```python
from build123d import *

# Parameters (mm, degrees)
F0_R     = 9.5
F0_R_2   = 4.1
F0_R_3   = 1.9
F1_DEPTH = 2
F2_R     = 4.1
F2_R_2   = 1.9
F3_DEPTH = 5.5
F4_R     = 1.5
F7_DEPTH = 7


# Not quite as in the source:
# - a feature names something its author has since deleted; it is built from what else it names


with BuildPart() as f1:
    # F0 (on Top) → F1 (new body)
    with BuildSketch(Plane.XY):
        Circle(F0_R)
        Circle(F0_R_2, mode=Mode.SUBTRACT)
        Circle(F0_R_2)
        Circle(F0_R_3, mode=Mode.SUBTRACT)
        Circle(F0_R_3)
    extrude(amount=F1_DEPTH)

    # F2 (on Top) → F3 (join)
    with BuildSketch(Plane.XY):
        Circle(F2_R)
        Circle(F2_R_2, mode=Mode.SUBTRACT)
    extrude(amount=F3_DEPTH)

    # F4
    f4_edges = [f1.edges().sort_by_distance(p)[0] for p in [
        (-9.5, 0, 0),
    ]]
    fillet(f4_edges, radius=F4_R)

    # F5 (on Front) → F6 (revolve, cut)
    with BuildSketch(Plane.XZ):
        with BuildLine():
            ThreePointArc((0, 0), (23.1570723538, -9.489364109), (32.9962119038, -32.5))
            ThreePointArc((32.9962119038, -32.5), (23.510635891, -8.8429276462), (0, 1))
            Line((0, 1), (0, 0))
        make_face()
    revolve(axis=Axis((0, 0, -31.5146126637), (0, 0, -1)), mode=Mode.SUBTRACT)

    # F7 (add): a face of the model
    f7_faces = [f1.faces().sort_by_distance(p)[0] for p in [
        (0, 0, 2),
    ]]
    extrude(f7_faces, amount=F7_DEPTH)


solid = f1.part
```
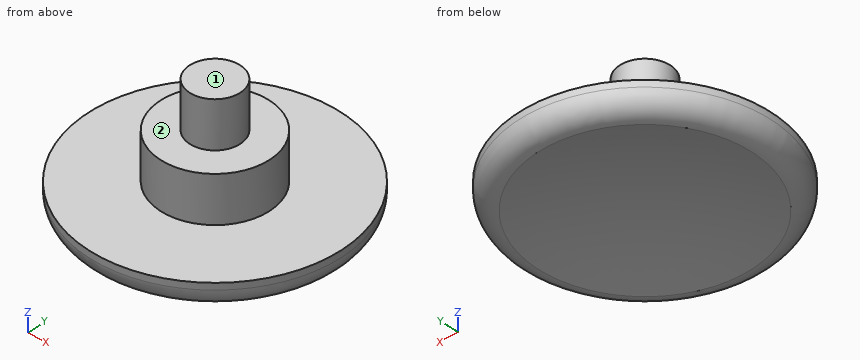
Input: part model. Units: mm. Frame: model coordinates. Face numbers are marked on the shaded views. A direction names the side the tool comes from. Give positions to 0.01 mm unless a question says otherwise; leave off trailing zeros. Write each loop counter-clockwise with the first axis right and the second up, starting at its lowest first coordinate (ties: lowest second). Pieces come first, ordered by that corner, then holes. Notation, with made-up numbers: (-32.75, -35.75) - (19.25, -35.75) arc R18 ccw to (19.25, -23.75) - close; hole circle Ø9 at (-5, 19). An arc over 180 degrees is marked (long way). Write item = value, one per line. Start each with the question number.
1) Reachability of the marked faces 1 and 2 from +Z, -Z, +X, -X, +Y, -Y: full face, straight path, thin tool, end or side. Return the list, or none.
2) Pin query (flat end, axial travel): pin 1 (4 mm diameter, centred on x = -6, y = -1.5, fed in from +Z); pin 2 (8 mm diameter, centred on x = -6, y = 0, fed in from +Z); pin 3 (1 mm diameter, centred on x = 3, y = 0, fed in from -Z). Return the tip coordinate at first contact, or that it passes through.
3) Cut plane B-B (z = 1.75). Return loops of the section in (x, y), and give its area (3 significant figures).
4) Cut plane A-A (y = 0). Return loops of the section in (x, z).
5) Material intervals for L1, parallel to Y at x = 5, z = 1.25; L2, parallel to Y at x = 0, z = 6.5; L3, parallel to Z at x = -2, y = -7, sorted ascending. Write a range as [from, to].
6) Cut plane C-C (z = 4.75). Return loops of the section in (x, y).
Answers follow:
q1.face_1 = +Z, +X, -X, +Y, -Y
q1.face_2 = +Z
q2.pin_1 = 2
q2.pin_2 = 5.5
q2.pin_3 = 0.81
q3.outline = circle Ø19 at (0, 0)
q3.area = 284 mm^2
q4.outline = (-9.5, 1.5) arc R1.5 ccw to (-8.06, 0) arc R33 cw to (8.06, 0) arc R1.5 ccw to (9.5, 1.5) - (9.5, 2) - (4.1, 2) - (4.1, 5.5) - (1.9, 5.5) - (1.9, 9) - (-1.9, 9) - (-1.9, 5.5) - (-4.1, 5.5) - (-4.1, 2) - (-9.5, 2) - close
q5.L1 = [-8.05, 8.05]
q5.L2 = [-1.9, 1.9]
q5.L3 = [0.19, 2]
q6.outline = circle Ø8.2 at (0, 0)
